from build123d import *

# Parameters (mm, degrees)
SKETCH1_R           = 1.7272
BOSS_EXTRUDE1_DEPTH = 5.9055
SKETCH2_R           = 10.31875
BOSS_EXTRUDE2_DEPTH = 28.575
SKETCH3_R           = 8.1534
CUT_EXTRUDE1_DEPTH  = 7.62
SKETCH4_R           = 6.7945
CUT_EXTRUDE2_DEPTH  = 16.256
SKETCH5_R           = 5.08
CUT_EXTRUDE3_DEPTH  = 40.987435874


with BuildPart() as part:
    # Sketch1 → Boss-Extrude1 (new body)
    with BuildSketch(Plane(origin=(0, 0, 0), x_dir=(1, 0, 0), z_dir=(0, 1, 0))):
        with BuildLine():
            Line((-15.0296372, 2.004639139), (-9.6266, 8.283632805))
            ThreePointArc((-9.6266, 8.283632805), (0, 12.7), (9.6266, 8.283632805))
            Line((9.6266, 8.283632805), (15.0296372, 2.004639139))
            ThreePointArc((15.0296372, 2.004639139), (15.7734, 0), (15.0296372, -2.004639139))
            Line((15.0296372, -2.004639139), (9.6266, -8.283632805))
            ThreePointArc((9.6266, -8.283632805), (0, -12.7), (-9.6266, -8.283632805))
            Line((-9.6266, -8.283632805), (-15.0296372, -2.004639139))
            ThreePointArc((-15.0296372, -2.004639139), (-15.7734, 0), (-15.0296372, 2.004639139))
        make_face()
        with Locations(Location((-12.7, 0, 0), (0, 0, 270))):
            Circle(SKETCH1_R, mode=Mode.SUBTRACT)
        with Locations(Location((12.7, 0, 0), (0, 0, 270))):
            Circle(SKETCH1_R, mode=Mode.SUBTRACT)
    extrude(amount=BOSS_EXTRUDE1_DEPTH)

    # Sketch2 → Boss-Extrude2 (add)
    with BuildSketch(Plane.XZ):
        with Locations(Location((0, 0, 0), (0, 0, 90))):
            Circle(SKETCH2_R)
    extrude(amount=BOSS_EXTRUDE2_DEPTH)

    # Sketch3 → Cut-Extrude1 (cut)
    with BuildSketch(Plane(origin=(0, 5.9055, 0), x_dir=(1, 0, 0), z_dir=(0, 1, 0))):
        with Locations(Location((0, 0, 0), (0, 0, 270))):
            Circle(SKETCH3_R)
    extrude(amount=-CUT_EXTRUDE1_DEPTH, mode=Mode.SUBTRACT)

    # Sketch4 → Cut-Extrude2 (cut)
    with BuildSketch(Plane(origin=(0, 5.9055, 0), x_dir=(1, 0, 0), z_dir=(0, 1, 0))):
        with Locations(Location((0, 0, 0), (0, 0, 270))):
            Circle(SKETCH4_R)
    extrude(amount=-CUT_EXTRUDE2_DEPTH, mode=Mode.SUBTRACT)

    # Sketch5 → Cut-Extrude3 (cut, through all)
    with BuildSketch(Plane(origin=(0, 5.9055, 0), x_dir=(1, 0, 0), z_dir=(0, 1, 0))):
        with Locations(Location((0, 0, 0), (0, 0, 270))):
            Circle(SKETCH5_R)
    extrude(amount=-CUT_EXTRUDE3_DEPTH, mode=Mode.SUBTRACT)


solid = part.part
The listing builds one solid part. Answer for the finished solid, in the listing's coordinates (mm). A direction names the side the tool comes from. Round coordinates to 2 decimals unless told otherwise and drop trailing zeros. Loops run counter-clockwise (first coordinate to the right, second up) from the corner with the lowest first, then second, coordinate; pieces in that order, holes last. Notation, with made-up numbers: M 16.25,3.25 L 44.25,3.25 A7 cw 44.25,14.25 Z; hole C 25,27.25 d11. An arc over 180 degrees is marked long. Return JSON: item names as keys, results as strings.
Q1. Find section A-A, the plane x = 0. Determine the outline of the cut face in (y, z) (1 decimal), plus the area to 3 significant figures.
Results list:
{"outline": "M -28.6,-10.3 L 0,-10.3 L 0,-12.7 L 5.9,-12.7 L 5.9,-8.2 L -1.7,-8.2 L -1.7,-6.8 L -10.4,-6.8 L -10.4,-5.1 L -28.6,-5.1 Z; M -28.6,5.1 L -10.4,5.1 L -10.4,6.8 L -1.7,6.8 L -1.7,8.2 L 5.9,8.2 L 5.9,12.7 L 0,12.7 L 0,10.3 L -28.6,10.3 Z", "area": "313 mm2"}
Q2. Each of these flat-tipped pins is pushed along its axis until it touches: pin 1 Ø3 at (y, z) = (-13, 0) entering from +X; pin 2 Ø3 at (x, z) = (-12.7, 0) entering from -Y; pin 3 Ø1.5 at (x, y) = (8, -2.5) entering from +Z; pin 4 Ø3 at (y, z) = (-12.5, 8) entering from -X. Where does it stop, or does it pass through?
Results list:
{"pin 1": "stops at x = 10.32", "pin 2": "passes through", "pin 3": "stops at z = 7.34", "pin 4": "stops at x = -8.01"}
Q3. The mould has two halves that part along Z. Classify faces 1 (the face through (15.773, 2.911, -0.031)), 2 (the face through (7, -1.715, -2)), 3 (the face through (2.4, 0, 10.3)): released by +Z, released by -Z, zero draft, split by the parting line, or undercut.
Results list:
{"face 1": "split by the parting line", "face 2": "undercut", "face 3": "zero draft"}
Q4. Find the intervals of material crossed by line 1 along X through (y, z) = (-21.75, 0); line 2 along X through (y, z) = (-2.5, 0); line 3 along Y through (x, z) = (-7, -1) (1 decimal), in increasing order. Write a range as from..to.
Results list:
{"line 1": "x = -10.32..-5.08, 5.08..10.32", "line 2": "x = -10.32..-6.79, 6.79..10.32", "line 3": "y = -28.6..-1.7"}
Q5. Which of the six approach directions +Z, -Z, +X, -X, +Y, -Y give full straight-line access (tool end or side, diameter ignored) to faces 4 (the face through (11.014, 2.911, -0.374)), 5 (the face through (-2.602, -5.972, 6.276)), 6 (the face through (-10.23, -14.09, -1.34))?
Results list:
{"face 4": "+Y, -Y", "face 5": "+Y", "face 6": "-Y"}
Q6. Find section D-D, the plane y = -4.5. Determine the outline of the cut face in (x, z).
Results list:
{"outline": "C 0,0 d20.64; hole C 0,0 d13.59"}
Q7. Find section B-B, the plane z = 0. Determine the outline of the cut face in (x, y) (1 decimal).
Results list:
{"outline": "M -15.8,0 L -14.4,0 L -14.4,5.9 L -15.8,5.9 Z; M -11,0 L -10.3,0 L -10.3,-28.6 L -5.1,-28.6 L -5.1,-10.4 L -6.8,-10.4 L -6.8,-1.7 L -8.2,-1.7 L -8.2,5.9 L -11,5.9 Z; M 5.1,-28.6 L 10.3,-28.6 L 10.3,0 L 11,0 L 11,5.9 L 8.2,5.9 L 8.2,-1.7 L 6.8,-1.7 L 6.8,-10.4 L 5.1,-10.4 Z; M 14.4,0 L 15.8,0 L 15.8,5.9 L 14.4,5.9 Z"}
Q8. Find section C-C, the plane z = -4. Determine the outline of the cut face in (x, y) (1 decimal), plus the area to 3 significant figures.
Results list:
{"outline": "M -13.3,0 L -9.5,0 L -9.5,-28.6 L -3.1,-28.6 L -3.1,-10.4 L -5.5,-10.4 L -5.5,-1.7 L -7.1,-1.7 L -7.1,5.9 L -13.3,5.9 Z; M 3.1,-28.6 L 9.5,-28.6 L 9.5,0 L 13.3,0 L 13.3,5.9 L 7.1,5.9 L 7.1,-1.7 L 5.5,-1.7 L 5.5,-10.4 L 3.1,-10.4 Z", "area": "384 mm2"}
